```python
from build123d import *
from OCP.BRepFilletAPI import BRepFilletAPI_MakeChamfer

# Parameters (mm, degrees)
BOSS_EXTRUDE1_DEPTH = 2.29
SKETCH3_W           = 0.64
SKETCH3_H           = 0.64
CHAMFER3_SIZE       = 0.5
CHAMFER3_SIZE2      = 0.133974596


with BuildPart() as part:
    # Sketch1 → Boss-Extrude1 (new body)
    with BuildSketch(Plane(origin=(0, 0, 0), x_dir=(1, 0, 0), z_dir=(0, 1, 0))):
        Polygon((-0.77, 1.25), (0.77, 1.25), (1.25, 0.75), (1.27, 0.75), (1.27, -0.75), (1.25, -0.75), (0.77, -1.25), (-0.77, -1.25), (-1.25, -0.75), (-1.27, -0.75), (-1.27, 0.75), (-1.25, 0.75), align=None)
    extrude(amount=BOSS_EXTRUDE1_DEPTH)

    # Sweep1: sweep along a path in Sketch2
    with BuildLine(Plane(origin=(0, 0, 0), x_dir=(0, 0, -1), z_dir=(1, 0, 0))) as sweep1_path:
        Line((0, 17.12), (0, -0.408142235))
        ThreePointArc((0, -0.408142235), (-0.152240935, -1.1735091), (-0.585786438, -1.822355798))
        Line((-0.585786438, -1.822355798), (-5.26343064, -6.5))
    # Sketch3 → Sweep1 (sweep)
    with BuildSketch(Plane(origin=(0, 17.12, 0), x_dir=(1, 0, 0), z_dir=(0, 1, 0))):
        Rectangle(SKETCH3_W, SKETCH3_H)
    sweep(path=sweep1_path.line)

    # Chamfer3: one chamfer whose edges measure the first distance from different faces: ONE call of the kernel's chamfer builder (chamfer() names one face for all edges)
    chamfer3_edges_1 = [part.edges().sort_by_distance(p)[0] for p in [
        (0.32, 17.12, 0),
    ]]
    chamfer3_side_1 = [part.faces().sort_by_distance(p)[0] for p in [
        (0.32, 9.705, 0),
    ]]
    chamfer3_edges_2 = [part.edges().sort_by_distance(p)[0] for p in [
        (0, 17.12, -0.32),
    ]]
    chamfer3_side_2 = [part.faces().sort_by_distance(p)[0] for p in [
        (0, 9.705, -0.32),
    ]]
    chamfer3_edges_3 = [part.edges().sort_by_distance(p)[0] for p in [
        (-0.32, 17.12, 0),
    ]]
    chamfer3_side_3 = [part.faces().sort_by_distance(p)[0] for p in [
        (-0.32, 9.705, 0),
    ]]
    chamfer3_edges_4 = [part.edges().sort_by_distance(p)[0] for p in [
        (0, 17.12, 0.32),
    ]]
    chamfer3_side_4 = [part.faces().sort_by_distance(p)[0] for p in [
        (0, 9.705, 0.32),
    ]]
    chamfer3 = BRepFilletAPI_MakeChamfer(part.part.solid().wrapped)
    for e in chamfer3_edges_1:
        chamfer3.Add(CHAMFER3_SIZE, CHAMFER3_SIZE2, e.wrapped, chamfer3_side_1[0].wrapped)  # the first distance lies on this face
    for e in chamfer3_edges_2:
        chamfer3.Add(CHAMFER3_SIZE, CHAMFER3_SIZE2, e.wrapped, chamfer3_side_2[0].wrapped)  # the first distance lies on this face
    for e in chamfer3_edges_3:
        chamfer3.Add(CHAMFER3_SIZE, CHAMFER3_SIZE2, e.wrapped, chamfer3_side_3[0].wrapped)  # the first distance lies on this face
    for e in chamfer3_edges_4:
        chamfer3.Add(CHAMFER3_SIZE, CHAMFER3_SIZE2, e.wrapped, chamfer3_side_4[0].wrapped)  # the first distance lies on this face
    add(Compound.cast(chamfer3.Shape()), mode=Mode.REPLACE)


solid = part.part
```
Design review of the part built by this model. Coordinates are the model's own, in mm. A direction names the side the tool comes from. Coordinates: 2 decimals unless noted, no trailing zeros. Order: outer loops, then holes, each group sorted by start corner. A loop starts at its lowest first (then second) coordinate and runs counter-clockwise, first axis right, second up. Notation, with made-up numbers: M 77,64 L 136,64 A19 ccw 136,81 Z; hole C 62,34.5 d10. An arc over 180 degrees is marked long. Answer as a JSON object with one key per item and string values. Group by question number.
1) Add section A-A, the plane x = 0.55. Write out the cut boundary in (y, z).
2) Tool access review of faces 1 (the flat face through (0, 0, -1)), 2 (the flat face through (0.32, -3, 2)), 3 (the flat face through (0, 1, 1.25)): name each direction out of +Z, -Z, +X, -X, +Y, -Y from which nothing blocks a thin tool from reaching the whole face with its end or side.
3) Add section B-B, the plane y = 8. Write out the cut boundary in (x, z), then the cut area to 3 significant figures.
4) Wall thickness on L1, parallel to Y at x = 0.8, z = 0.5; L2, parallel to X at y = 8.5, z = -0.25: over which ranges is each line inside the solid? List them lowest first.
5) For pin 1 (0.5 mm diameter, centred on y = 9, z = 0, fed in from -X); pin 2 (1.2 mm diameter, centred on x = 0.5, z = 0.5, fed in from -Y); pin 3 (0.7 mm diameter, centred on x = 0, y = 6, fed in from -Z); pin 4 (1.5 mm diameter, centred on y = -4, z = 0.5, fed in from -X), all flat-tipped, find the tip position at first contact; note any pin that passes through.
Computed values:
{
 "1": {"outline": "M 0,-1.25 L 2.29,-1.25 L 2.29,1.25 L 0,1.25 Z"},
 "2": {"face 1": "none", "face 2": "+Z, -Z, +X, -Y", "face 3": "+Z, +X, -X, +Y"},
 "3": {"outline": "M -0.32,-0.32 L 0.32,-0.32 L 0.32,0.32 L -0.32,0.32 Z", "area": "0.410 mm^2"},
 "4": {"L1": "y = 0 to 2.29", "L2": "x = -0.32 to 0.32"},
 "5": {"pin 1": "stops at x = -0.32", "pin 2": "stops at y = -2.76", "pin 3": "stops at z = -0.32", "pin 4": "passes through"}
}
